CAD build for the part. Positions are in the model's coordinates, mm. A direction names the side the tool comes from. Give positions to 0.01 mm unless a question says otherwise; leave off trailing zeros. Order: outer loops, then holes, each group sorted by start corner. A loop starts at its lowest first (then second) coordinate and runs counter-clockwise, first axis right, second up.
from build123d import *

# Parameters (mm, degrees)
SKETCH1_R                           = 9.05
SKETCH1_R_2                         = 7.5565
PLATE_DEPTH                         = 3.81
SKETCH1_3_R                         = 7.5565
PLUG_DEPTH                          = 17.78
CUT_EXTRUDE1_REACH                  = 23.907
CUT_EXTRUDE1_END_RADIUS             = 7.5565
SKETCH4_R                           = 2.0955
CUT_EXTRUDE1_DIRECTION_2_REACH      = 23.907
CUT_EXTRUDE1_DIRECTION_2_END_RADIUS = 7.5565
FILLET1_R                           = 0.762
CUT_EXTRUDE2_REACH                  = 23.907
SKETCH5_R                           = 2.9845


with BuildPart() as part:
    # Sketch1 → Plate (new body)
    # profile 1 of 2: a face of its own
    with BuildSketch(Plane(origin=(0, 0, 0), x_dir=(1, 0, 0), z_dir=(0, 1, 0))):
        with Locations(Location((0, 0, 0), (0, 0, 90))):
            Circle(SKETCH1_R)
        Circle(SKETCH1_R_2, mode=Mode.SUBTRACT)
    # profile 2 of 2: a face of its own
    with BuildSketch(Plane(origin=(0, 0, 0), x_dir=(1, 0, 0), z_dir=(0, 1, 0))):
        Circle(SKETCH1_R_2)
    extrude(amount=PLATE_DEPTH)

    # Sketch1_3 → Plug (add)
    with BuildSketch(Plane(origin=(0, 0, 0), x_dir=(1, 0, 0), z_dir=(0, 1, 0))):
        with Locations(Location((0, 0, 0), (0, 0, 270))):
            Circle(SKETCH1_3_R)
    extrude(amount=PLUG_DEPTH)

    # Cut-Extrude1: up to this cylinder (the profile starts inside it)
    cut_extrude1_end = Plane(origin=(0, 10.922, 0), z_dir=(0, -1, 0)) * Cylinder(CUT_EXTRUDE1_END_RADIUS, 63.927, mode=Mode.PRIVATE)
    # Sketch4 → Cut-Extrude1 (cut, up to the surface)
    with BuildSketch(Plane(origin=(0, 0, 0), x_dir=(0, 0, -1), z_dir=(1, 0, 0)), mode=Mode.PRIVATE) as cut_extrude1_sk1:
        with Locations((0, 10.922)):
            Circle(SKETCH4_R)
    cut_extrude1_tool1 = extrude(cut_extrude1_sk1.sketch, amount=-CUT_EXTRUDE1_REACH, mode=Mode.PRIVATE) & cut_extrude1_end
    add(cut_extrude1_tool1.solids().sort_by_distance((0, 10.922, 0))[0], mode=Mode.SUBTRACT)

    # Cut-Extrude1 direction 2: up to this cylinder (the profile starts inside it)
    cut_extrude1_direction_2_end = Plane(origin=(0, 10.922, 0), z_dir=(0, -1, 0)) * Cylinder(CUT_EXTRUDE1_DIRECTION_2_END_RADIUS, 63.927, mode=Mode.PRIVATE)
    # Sketch4 → Cut-Extrude1 direction 2 (cut, up to the surface)
    with BuildSketch(Plane(origin=(0, 0, 0), x_dir=(0, 0, -1), z_dir=(1, 0, 0)), mode=Mode.PRIVATE) as cut_extrude1_direction_2_sk1:
        with Locations((0, 10.922)):
            Circle(SKETCH4_R)
    cut_extrude1_direction_2_tool1 = extrude(cut_extrude1_direction_2_sk1.sketch, amount=CUT_EXTRUDE1_DIRECTION_2_REACH, mode=Mode.PRIVATE) & cut_extrude1_direction_2_end
    add(cut_extrude1_direction_2_tool1.solids().sort_by_distance((0, 10.922, 0))[0], mode=Mode.SUBTRACT)

    # Fillet1
    fillet1_edges = [part.edges().sort_by_distance(p)[0] for p in [
        (0, 17.78, -7.5565),
    ]]
    fillet(fillet1_edges, radius=FILLET1_R)

    # Sketch5 → Cut-Extrude2 (cut, up to next)
    with BuildSketch(Plane(origin=(0, 17.78, 0), x_dir=(1, 0, 0), z_dir=(0, 1, 0)), mode=Mode.PRIVATE) as cut_extrude2_sk1:
        with Locations(Location((0, 0, 0), (0, 0, 270))):
            Circle(SKETCH5_R)
    cut_extrude2_tool1 = extrude(cut_extrude2_sk1.sketch, amount=-CUT_EXTRUDE2_REACH, mode=Mode.PRIVATE) & part.part
    add(cut_extrude2_tool1.solids().sort_by_distance((0, 17.78, 0))[0], mode=Mode.SUBTRACT)


solid = part.part
1. Wall check: line 1 (Y direction, x = -4.05, z = 0); line 2 (Y direction, x = 7.5, z = -1.75); line 3 (X direction, y = 14.75, z = 0.5). Give the ranges that are in metal, low to high.
2. Saw through at C-C on y = 12.75. Give the cut face in (x, z).
3. 3-axis set-ups, long thin cutter, end or side, ignore diameter. For faces 5 (the cylindrical face through (2.3, 10.3, 7.2)), 6 (the flat face through (-4, 0, 0)): which of +Z, -Z, +X, -X, +Y, -Y reach the whole face in a straight line?
4. Saw through at B-B on z = 0. Give the cut face in (x, y), plus the area to 3 significant figures.
5. Mould opens along Z. For faces 1 (the flat face through (-1, 17.78, 3)), 2 (the cylindrical face through (4.81, 11.55, -2)), 3 (the cylindrical face through (-4.81, 11.55, -2)), 4 (the cylindrical face through (-2.72, 1.88, -8.63)) say: released by +Z, released by -Z, zero draft, split by the parting line, or undercut.
6. Pin check, flat tips, straight feed: P1, Ø4, axis at y = 6.5, z = 5, coming from the -X side; P2, Ø10, axis at x = 7, z = 2, coming from the +Y side; P3, Ø5, axis at y = 10.922, z = 0, coming from the +X side; P4, Ø5.5, axis at y = 10.922, z = 0, coming from the -X side. Stop position of each tip, or through.
7. Saw through at A-A on x = 0. Give the cut face in (y, z).
Reported:
1. line 1: y = 0 to 8.83, 13.02 to 17.78
1. line 2: y = 0 to 3.81
1. line 3: x = -7.54 to -2.94, 2.94 to 7.54
2. outline: (-7.49, -1.02) arc R7.56 ccw to (7.49, -1.02) - (2.8, -1.02) arc R2.98 cw to (-2.8, -1.02) - close; (-7.49, 1.02) - (-2.8, 1.02) arc R2.98 cw to (2.8, 1.02) - (7.49, 1.02) arc R7.56 ccw to start
3. face 5: +Y
3. face 6: +Z, -Z, +X, -X, -Y
4. outline: (-9.05, 0) - (-2.98, 0) - (-2.98, 8.83) - (-7.56, 8.83) - (-7.56, 3.81) - (-9.05, 3.81) - close; (-7.56, 13.02) - (-2.98, 13.02) - (-2.98, 17.78) - (-6.79, 17.78) arc R0.76 ccw to (-7.56, 17.02) - close; (2.98, 0) - (9.05, 0) - (9.05, 3.81) - (7.56, 3.81) - (7.56, 8.83) - (2.98, 8.83) - close; (2.98, 13.02) - (7.56, 13.02) - (7.56, 17.02) arc R0.76 ccw to (6.79, 17.78) - (2.98, 17.78) - close
4. area: 135 mm2
5. face 1: zero draft
5. face 2: undercut
5. face 3: undercut
5. face 4: split by the parting line
6. P1: stops at x = -6.94
6. P2: stops at y = 17.78
6. P3: stops at x = 7.56
6. P4: stops at x = -7.56
7. outline: (0, -9.05) - (3.81, -9.05) - (3.81, -7.56) - (17.02, -7.56) arc R0.76 ccw to (17.78, -6.79) - (17.78, -2.98) - (0, -2.98) - close; (0, 2.98) - (17.78, 2.98) - (17.78, 6.79) arc R0.76 ccw to (17.02, 7.56) - (3.81, 7.56) - (3.81, 9.05) - (0, 9.05) - close
